from build123d import *

# Parameters (mm, degrees)
BASE_FLANGE1_DEPTH = 10
FILLET1_R          = 0.9
SKETCH6_R          = 2.5
CUT_EXTRUDE3_DEPTH = 21.615528128
SKETCH7_R          = 2.5
CUT_EXTRUDE4_DEPTH = 22.066798523
SKETCH8_R          = 2.5
CUT_EXTRUDE5_DEPTH = 26.605077621


# Sheet-metal steps are written as plain solids
with BuildPart() as part:
    # Sketch1 → Base-Flange1 (new body)
    with BuildSketch(Plane.XY):
        with BuildLine():
            Line((-4.1, 10), (4.1, 10))
            ThreePointArc((4.1, 10), (4.736396103, 9.736396103), (5, 9.1))
            Line((5, 9.1), (5, 0.9))
            ThreePointArc((5, 0.9), (5.263603897, 0.263603897), (5.9, 0))
            Line((5.9, 0), (15, 0))
            Line((15, 0), (15, 0.9))
            Line((15, 0.9), (5.9, 0.9))
            Line((5.9, 0.9), (5.9, 9.1))
            ThreePointArc((5.9, 9.1), (5.372792206, 10.372792206), (4.1, 10.9))
            Line((4.1, 10.9), (-4.1, 10.9))
            ThreePointArc((-4.1, 10.9), (-5.372792206, 10.372792206), (-5.9, 9.1))
            Line((-5.9, 9.1), (-5.9, 0.9))
            Line((-5.9, 0.9), (-15, 0.9))
            Line((-15, 0.9), (-15, 0))
            Line((-15, 0), (-5.9, 0))
            ThreePointArc((-5.9, 0), (-5.263603897, 0.263603897), (-5, 0.9))
            Line((-5, 0.9), (-5, 9.1))
            ThreePointArc((-5, 9.1), (-4.736396103, 9.736396103), (-4.1, 10))
        make_face()
    extrude(amount=-BASE_FLANGE1_DEPTH)

    # Fillet1
    fillet1_edges = [part.edges().sort_by_distance(p)[0] for p in [
        (-5.9, 0.9, -5),
        (5.9, 0.9, -5),
    ]]
    fillet(fillet1_edges, radius=FILLET1_R)

    # Sketch6 → Cut-Extrude3 (cut, through all)
    with BuildSketch(Plane(origin=(0, 0.9, 0), x_dir=(1, 0, 0), z_dir=(0, 1, 0))):
        with Locations(Location((-10, 5, 0), (0, 0, 180))):
            Circle(SKETCH6_R)
        with BuildLine():
            Line((-15, 10), (-15, 5))
            ThreePointArc((-15, 5), (-13.535533906, 8.535533906), (-10, 10))
            Line((-10, 10), (-15, 10))
        make_face()
        with BuildLine():
            Line((-15, 0), (-10, 0))
            ThreePointArc((-10, 0), (-13.535533906, 1.464466094), (-15, 5))
            Line((-15, 5), (-15, 0))
        make_face()
    cut_extrude3 = extrude(amount=-CUT_EXTRUDE3_DEPTH, mode=Mode.SUBTRACT)

    # Mirror1: Cut-Extrude3 across plane
    add(cut_extrude3.mirror(Plane(origin=(0, 0, 0), x_dir=(0, 0, 1), z_dir=(1, 0, 0))), mode=Mode.SUBTRACT)

    # Sketch7 → Cut-Extrude4 (cut, through all)
    with BuildSketch(Plane(origin=(0, 10.9, 0), x_dir=(1, 0, 0), z_dir=(0, 1, 0))):
        with Locations(Location((0, 5, 0), (0, 0, 180))):
            Circle(SKETCH7_R)
    extrude(amount=-CUT_EXTRUDE4_DEPTH, mode=Mode.SUBTRACT)

    # Sketch8 → Cut-Extrude5 (cut, through all)
    with BuildSketch(Plane(origin=(5.9, 0, 0), x_dir=(0, 0, -1), z_dir=(1, 0, 0))):
        with Locations(Location((5, 5, 0), (0, 0, 90))):
            Circle(SKETCH8_R)
    extrude(amount=-CUT_EXTRUDE5_DEPTH, mode=Mode.SUBTRACT)


solid = part.part
Geometry: final body of the model. Coordinates: model frame, mm. A direction names the side the tool comes from. Round coordinates to 2 decimals unless told otherwise and drop trailing zeros. Loops run counter-clockwise (first coordinate to the right, second up) from the corner with the lowest first, then second, coordinate; pieces in that order, holes last. Notation, with made-up numbers: (59.5, -12) -> (105.5, -12) arc R37 ccw to (105.5, 26) -> close; hole circle Ø5 at (84, 84.5). An arc over 180 degrees is marked (long way). One line per question, with ' | ' between items. Start each with the question number.
1. Line query: line 1 along X through (y, z) = (5, -7.75); line 2 along Z through (x, y) = (5.6, 5); line 3 along Y through (x, z) = (3.25, -3.5). Output: solid intervals per line, ascending. Write a range as [from, to].
2. Section A-A on x = 0. Output: boundary loops of the cut face in (y, z), and give its area (3 significant figures).
3. Mould query, pull axis X, two halves, no side actions, for faces 4 (the face through (-5, 2, -5)), 5 (the face through (13, 0.9, -5)), 6 (the face through (-6.16, 1.17, -5.07)). Classes: pulls with the +X half, pulls with the -X half, needs draft (parallel to the pull), parting line crosses it, or undercut.
4. Contact query for flat-ended pins moving along their axis: pin 1 (4 mm diameter, centred on x = -9, z = -3, fed in from +Y); pin 2 (3 mm diameter, centred on y = 9.5, z = -6, fed in from +X); pin 3 (2 mm diameter, centred on y = 7, z = -4.5, fed in from -X); pin 4 (6 mm diameter, centred on x = 0, y = 6, fed in from +Z). Output: stop coordinate, or through.
5. Set-up query: faces 1 (the face through (-5.9, 8, -5)), 2 (the face through (5.9, 8, -5)), 3 (the face through (-4.74, 9.73, -4.93)). Return all of +Z, -Z, +X, -X, +Y, -Y with unobstructed straight access to the full face (end or side cutting, diameter ignored); none if empty.
6. Section D-D on z = -4. Count the separate pieces of the cut face and the enclosed holes in it, and give its area (3 significant figures).
7. Section C-C on y = 1.5. Output: boundary loops of the cut face in (x, z), and give its area (3 significant figures).
8. Section B-B on y = 5. Output: boundary loops of the cut face in (x, z), and give its area (3 significant figures).
Returned:
1) line 1: x = [-5.9, -5], [5, 5.9] | line 2: z = [-10, -7.5], [-2.5, 0] | line 3: y = [10, 10.9]
2) outline: (10, -10) -> (10.9, -10) -> (10.9, -7.5) -> (10, -7.5) -> close; (10, -2.5) -> (10.9, -2.5) -> (10.9, 0) -> (10, 0) -> close | area: 4.50 mm2
3) face 4: undercut | face 5: needs draft | face 6: pulls with the -X half
4) pin 1: stops at y = 0.9 | pin 2: stops at x = 5.9 | pin 3: stops at x = -5.9 | pin 4: passes through
5) face 1: +Z, -Z, -X, +Y | face 2: +Z, -Z, +X, +Y | face 3: +Z, -Z, -Y
6) separate pieces: 6 | enclosed holes: 0 | area: 23.2 mm2
7) outline: (-5.95, -10) -> (-5, -10) -> (-5, 0) -> (-5.95, 0) -> close; (5, -10) -> (5.95, -10) -> (5.95, 0) -> (5, 0) -> close | area: 19.0 mm2
8) outline: (-5.9, -10) -> (-5, -10) -> (-5, -7.5) -> (-5.9, -7.5) -> close; (-5.9, -2.5) -> (-5, -2.5) -> (-5, 0) -> (-5.9, 0) -> close; (5, -10) -> (5.9, -10) -> (5.9, -7.5) -> (5, -7.5) -> close; (5, -2.5) -> (5.9, -2.5) -> (5.9, 0) -> (5, 0) -> close | area: 9.00 mm2
